Study the drawing (mm; zero at the part's minimum x, y, z) and answer. A direction names the side the tool comes from. Give positions to 0.01 mm unless a question says otherwise; leave off trailing zeros. Write each loop counter-clockwise with the first axis right and the second up, starting at its lowest first coordinate (ties: lowest second). Pieces come first, ordered by that corner, then holes. Notation, with made-up numbers: (66.5, 51) -> (106.5, 51) arc R32 cw to (106.5, 82) -> close; hole circle Ø3 at (65, 46.25). An arc over 180 degrees is marked (long way). Put each result on its own line as item: value. Start each with the question number.
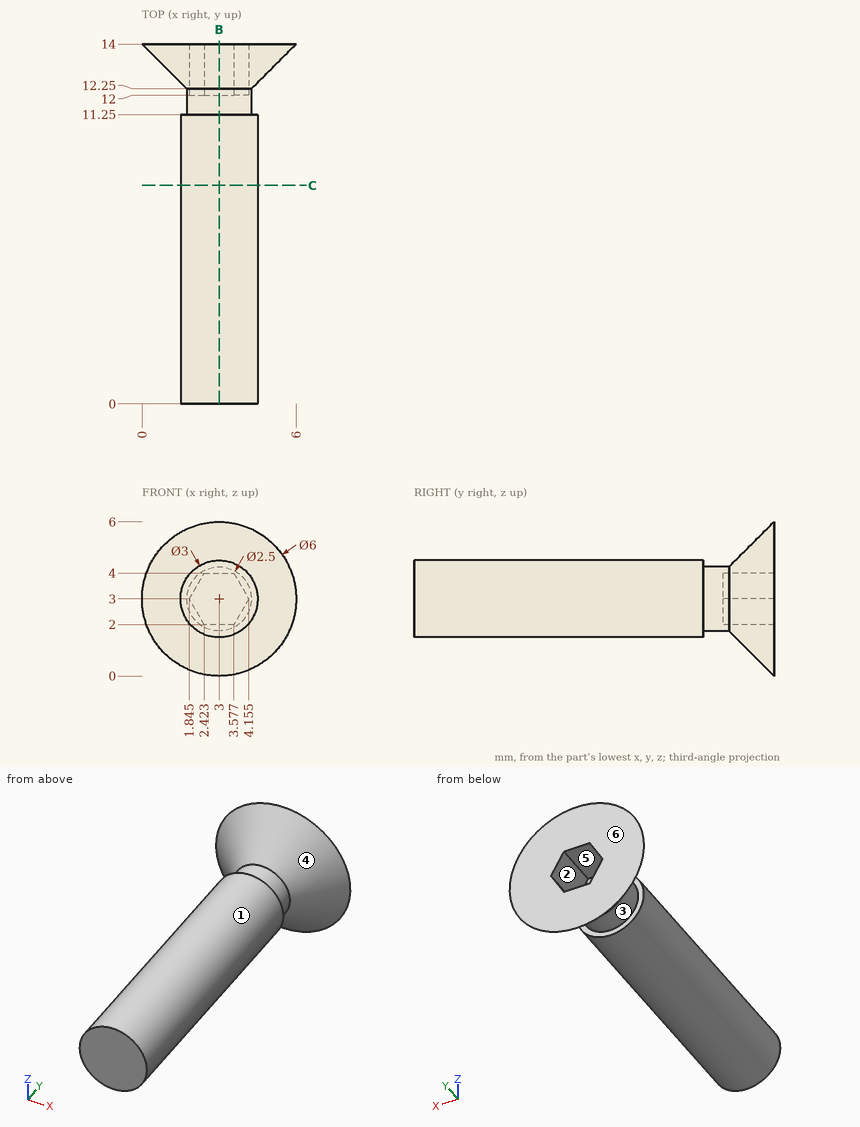
1) Each of these flat-tipped pins is pushed along its axis until it touches: pin 1 Ø1.5 at (x, y) = (5.5, 10) entering from -Z; pin 2 Ø2 at (x, y) = (2, 9) entering from -Z; pin 3 Ø2 at (x, y) = (3.5, 2.5) entering from +Z; pin 4 Ø1 at (x, y) = (1.5, 8.5) entering from +Z. Where does it stop, or does it pass through?
2) For a pull along Z with two mould halves and no side action, classify the marked faces 4, 5 and 6 as pulls with the +Z half, pulls with the -Z half, needs draft (parallel to the pull), parting line crosses it, or undercut.
3) For the marked faces 1, 2 and 3, determine the directions among +Z, -Z, +X, -X, +Y, -Y from which every point of the face is accessible in a straight line to the end or side of a thin tool.
4) Straight lines are drawn through the part: line 1 (X direction, y = 13.25, z = 2.4); line 2 (Y direction, x = 3, z = 3.8); line 3 (X direction, y = 4.25, z = 3.1). For each, find the intervals that lie inside material, in ascending order. Write a range as [from, to].
5) A cutting plane is placed at B-B on x = 3. Give the vertices of the cut face in (y, z), and give its area (3 significant figures).
6) A cutting plane is placed at C-C on y = 8.5. Give the vertices of the cut face in (x, z).
Results found:
1. pin 1: passes through
1. pin 2: stops at z = 1.5
1. pin 3: stops at z = 4.5
1. pin 4: stops at z = 4.12
2. face 4: parting line crosses it
2. face 5: undercut
2. face 6: needs draft
3. face 1: -Y
3. face 2: +Y
3. face 3: none
4. line 1: x = [0.83, 2.19], [3.81, 5.17]
4. line 2: y = [0, 12]
4. line 3: x = [1.5, 4.5]
5. outline: (0, 1.5) -> (11.25, 1.5) -> (11.25, 1.75) -> (12.25, 1.75) -> (14, 0) -> (14, 2) -> (12, 2) -> (12, 4) -> (14, 4) -> (14, 6) -> (12.25, 4.25) -> (11.25, 4.25) -> (11.25, 4.5) -> (0, 4.5) -> close
5. area: 39.7 mm²
6. outline: circle Ø3 at (3, 3)
